Source: CAD feature listing. Evaluate the final solid. Frame: model axes, mm. A direction names the side the tool comes from. Round coordinates to 2 decimals unless told otherwise and drop trailing zeros. Loops run counter-clockwise (first coordinate to the right, second up) from the corner with the lowest first, then second, coordinate; pieces in that order, holes last. Notation, with made-up numbers: (0, -30) -> (5, -30) arc R32 cw to (5, 4) -> close; hole circle Ø4 at (-3, 89). An arc over 180 degrees is marked (long way). Return JSON: item names as keys, results as strings. Group by question number.
```python
from build123d import *

# Parameters (mm, degrees)
F0_W      = 42
F0_H      = 14
F1_DEPTH  = 14
F3_DEPTH  = 25
F4_SIZE   = 3
F5_R      = 2
F6_DEPTH  = 25
F7_DEPTH  = 25
F8_W      = 10
F8_H      = 14
F9_DEPTH  = 10
F10_W     = 10
F10_H     = 10
F11_DEPTH = 7.5


with BuildPart() as f1:
    # F0 (on Top) → F1 (new body)
    with BuildSketch(Plane.XY):
        with Locations((21, -7)):
            Rectangle(F0_W, F0_H)
    extrude(amount=F1_DEPTH)

    # F2 (on face) → F3 (cut)
    with BuildSketch(Plane.XY.offset(14)):
        with BuildLine():
            ThreePointArc((37, -10.5), (38.06066, -10.06066), (38.5, -9))
            ThreePointArc((38.5, -9), (35.93934, -7.93934), (37, -10.5))
        make_face()
    extrude(amount=-F3_DEPTH, mode=Mode.SUBTRACT)

    # F4
    f4_edges = [f1.edges().sort_by_distance(p)[0] for p in [
        (0, -14, 7),
        (42, -14, 7),
    ]]
    chamfer(f4_edges, length=F4_SIZE)

    # F5 (on face) → F6 (cut)
    with BuildSketch(Plane(origin=(0, 0, 0), x_dir=(-1, 0, 0), z_dir=(0, 1, 0))):
        with BuildLine():
            ThreePointArc((-28, 7), (-27, 6), (-26, 7))
            ThreePointArc((-26, 7), (-27, 8), (-28, 7))
        make_face()
        with Locations((-10, 7)):
            Circle(F5_R)
    extrude(amount=-F6_DEPTH, mode=Mode.SUBTRACT)

    # F5 (on face) → F7 (cut)
    with BuildSketch(Plane(origin=(0, 0, 0), x_dir=(-1, 0, 0), z_dir=(0, 1, 0))):
        with BuildLine():
            ThreePointArc((-28, 7), (-27, 6), (-26, 7))
            ThreePointArc((-26, 7), (-27, 8), (-28, 7))
        make_face()
        with Locations((-10, 7)):
            Circle(F5_R)
    extrude(amount=-F7_DEPTH, mode=Mode.SUBTRACT)

    # F8 (on face) → F9 (join)
    with BuildSketch(Plane(origin=(0, 0, 0), x_dir=(-1, 0, 0), z_dir=(0, 1, 0))):
        with Locations((-37, 7)):
            Rectangle(F8_W, F8_H)
    extrude(amount=F9_DEPTH)

    # F10 (on face) → F11 (cut)
    with BuildSketch(Plane.XY.offset(14)):
        with Locations((37, 5)):
            Rectangle(F10_W, F10_H)
    extrude(amount=-F11_DEPTH, mode=Mode.SUBTRACT)


solid = f1.part
```
(1) Ray query, line 1 (Z direction, x = 10, y = -9.25); line 2 (X direction, y = -9, z = 8.5); line 3 (X direction, y = -5, z = 7.75). Return the intervals inside material, ascending.
(2) Cut plane A-A (z = 7). Return loops of the section in (x, y), and give its area (3 significant figures).
(3) Cut plane D-D (y = -4). Return loops of the section in (x, z), and give its area (3 significant figures).
(4) Mould query, pull axis Z, two halves, no side actions, for faces 3 (the face through (10, -7, 9)), 4 (the face through (37, 5, 6.5)), 5 (the face through (2, -13, 7)), 6 (the face through (26, -5, 0)). Classes: released by +Z, released by -Z, zero draft, split by the parting line, or undercut.
(5) Cut plane C-C (z = 11.5). Return loops of the section in (x, y), and give its area (3 significant figures).
(6) Pin query (flat end, axial travel): pin 1 (2 mm diameter, centred on x = 6, z = 6.5, fed in from +Y); pin 2 (11 mm diameter, centred on x = 39, y = 7.5, fed in from +Z); pin 3 (2 mm diameter, centred on y = 3, z = 4, fed in from -X). Return the tip coordinate at first contact, or that it passes through.
(7) Set-up query: faces 1 (the face through (41, -12, 7)), 2 (the face through (32, 5, 3)). Return all of +Z, -Z, +X, -X, +Y, -Y with unobstructed straight access to the full face (end or side cutting, diameter ignored); none if empty.
(8) Cut plane B-B (x = 10). Return loops of the section in (y, z), and give its area (3 significant figures).
Answers follow:
{
 "1": {"line 1": "0 to 5, 9 to 14", "line 2": "0 to 8.68, 11.32 to 35.5, 38.5 to 42", "line 3": "0 to 8.15, 11.85 to 26.34, 27.66 to 42"},
 "2": {"outline": "(0, -11) -> (3, -14) -> (8, -14) -> (8, 0) -> (0, 0) -> close; (12, -14) -> (26, -14) -> (26, 0) -> (12, 0) -> close; (28, -14) -> (39, -14) -> (42, -11) -> (42, 0) -> (28, 0) -> close; hole circle Ø3 at (37, -9)", "area": "488 mm^2"},
 "3": {"outline": "(0, 0) -> (42, 0) -> (42, 14) -> (0, 14) -> close; hole circle Ø4 at (10, 7); hole circle Ø2 at (27, 7)", "area": "572 mm^2"},
 "4": {"face 3": "undercut", "face 4": "released by +Z", "face 5": "zero draft", "face 6": "released by -Z"},
 "5": {"outline": "(0, -11) -> (3, -14) -> (39, -14) -> (42, -11) -> (42, 0) -> (0, 0) -> close; hole circle Ø3 at (37, -9)", "area": "572 mm^2"},
 "6": {"pin 1": "y = 0", "pin 2": "z = 6.5", "pin 3": "x = 32"},
 "7": {"face 1": "+Z, -Z, +X, -Y", "face 2": "+Z, -Z, -X, +Y"},
 "8": {"outline": "(-14, 0) -> (0, 0) -> (0, 5) -> (-14, 5) -> close; (-14, 9) -> (0, 9) -> (0, 14) -> (-14, 14) -> close", "area": "140 mm^2"}
}
